```python
from build123d import *

# Parameters (mm, degrees)
EXTRUDE_THIN1_DEPTH       = 100
BOSS_EXTRUDE1_START       = -10
BOSS_EXTRUDE1_DEPTH       = 10
SKETCH3_R                 = 2.25
BOSS_EXTRUDE2_DEPTH       = 5
BOSS_EXTRUDE3_DEPTH       = 10
SKETCH5_R                 = 2.25
CUT_EXTRUDE1_DEPTH        = 6
BOSS_EXTRUDE4_REACH       = 121.416
BOSS_EXTRUDE4_END_RADIUS  = 39
SKETCH10_W                = 20
SKETCH10_H                = 20
BOSS_EXTRUDE5_START       = -29.189050103
BOSS_EXTRUDE5_OUTLINE_W   = 20
BOSS_EXTRUDE5_OUTLINE_H   = 20
BOSS_EXTRUDE5_DEPTH       = 29.189050103
BOSS_EXTRUDE5_START_2     = 80.604897745
BOSS_EXTRUDE5_2_OUTLINE_W = 23
BOSS_EXTRUDE5_2_OUTLINE_H = 23
BOSS_EXTRUDE5_2_DEPTH     = 1.395102255
BOSS_EXTRUDE6_DEPTH       = 20
SKETCH12_R                = 2.5
CUT_EXTRUDE2_DEPTH        = 20


with BuildPart() as part:
    # Sketch1 → Extrude-Thin1 (new body)
    with BuildSketch(Plane.XY):
        with BuildLine():
            ThreePointArc((-35, 0), (0, -35), (35, 0))
            Line((35, 0), (39, 0))
            ThreePointArc((39, 0), (0, -39), (-39, 0))
            Line((-39, 0), (-35, 0))
        make_face()
    extrude(amount=EXTRUDE_THIN1_DEPTH)

    # Sketch2 → Boss-Extrude1 (add)
    with BuildSketch(Plane.XY.offset(100).offset(BOSS_EXTRUDE1_START)):
        with BuildLine():
            Line((0, -39), (0, -35))
            Line((0, -35), (-10, -35))
            Line((-10, -35), (-10, -37.69615365))
            ThreePointArc((-10, -37.69615365), (-5.042321274, -38.672664715), (0, -39))
        make_face()
        with BuildLine():
            Line((10, -35), (0, -35))
            Line((0, -35), (0, -39))
            ThreePointArc((0, -39), (5.042321274, -38.672664715), (10, -37.69615365))
            Line((10, -37.69615365), (10, -35))
        make_face()
        with BuildLine():
            ThreePointArc((10, -37.69615365), (5.042321274, -38.672664715), (0, -39))
            ThreePointArc((0, -39), (-5.042321274, -38.672664715), (-10, -37.69615365))
            Line((-10, -37.69615365), (-10, -43))
            Line((-10, -43), (10, -43))
            Line((10, -43), (10, -37.69615365))
        make_face()
    extrude(amount=BOSS_EXTRUDE1_DEPTH)

    # Sketch3 → Boss-Extrude2 (add)
    with BuildSketch(Plane.XY.offset(100)):
        with Locations((-5, -39)):
            Circle(SKETCH3_R)
        with Locations((5, -39)):
            Circle(SKETCH3_R)
    extrude(amount=BOSS_EXTRUDE2_DEPTH)

    # Sketch4 → Boss-Extrude3 (add)
    with BuildSketch(Plane(origin=(0, 0, 0), x_dir=(-1, 0, 0), z_dir=(0, 0, -1))):
        with BuildLine():
            Line((0, -39), (0, -35))
            Line((0, -35), (-10, -35))
            Line((-10, -35), (-10, -37.69615365))
            ThreePointArc((-10, -37.69615365), (-5.042321274, -38.672664715), (0, -39))
        make_face()
        with BuildLine():
            ThreePointArc((10, -37.69615365), (5.042321274, -38.672664715), (0, -39))
            ThreePointArc((0, -39), (-5.042321274, -38.672664715), (-10, -37.69615365))
            Line((-10, -37.69615365), (-10, -43))
            Line((-10, -43), (10, -43))
            Line((10, -43), (10, -37.69615365))
        make_face()
        with BuildLine():
            Line((10, -35), (0, -35))
            Line((0, -35), (0, -39))
            ThreePointArc((0, -39), (5.042321274, -38.672664715), (10, -37.69615365))
            Line((10, -37.69615365), (10, -35))
        make_face()
    extrude(amount=-BOSS_EXTRUDE3_DEPTH)

    # Sketch5 → Cut-Extrude1 (cut)
    with BuildSketch(Plane(origin=(0, 0, 0), x_dir=(-1, 0, 0), z_dir=(0, 0, -1))):
        with Locations(Location((-5, -39, 0), (0, 0, 180))):
            Circle(SKETCH5_R)
        with Locations(Location((5, -39, 0), (0, 0, 180))):
            Circle(SKETCH5_R)
    extrude(amount=-CUT_EXTRUDE1_DEPTH, mode=Mode.SUBTRACT)

    # Boss-Extrude4: up to this cylinder (the profile starts outside it)
    boss_extrude4_end = Plane(origin=(0, 0, 50), z_dir=(0, 0, -1)) * Cylinder(BOSS_EXTRUDE4_END_RADIUS, 321.832, mode=Mode.PRIVATE)
    # Sketch10 → Boss-Extrude4 (add, up to the surface)
    with BuildSketch(Plane(origin=(0, -51.355775573, 4.493048169), x_dir=(1, 0, 0), z_dir=(0, 0.9961946980917462, -0.08715574274765152)), mode=Mode.PRIVATE) as boss_extrude4_sk1:
        with Locations((0, -45.680780994)):
            Rectangle(SKETCH10_W, SKETCH10_H)
    boss_extrude4_tool1 = extrude(boss_extrude4_sk1.sketch, amount=BOSS_EXTRUDE4_REACH, mode=Mode.PRIVATE) - boss_extrude4_end
    add(boss_extrude4_tool1.solids().sort_by_distance((0, -47.374433, 50))[0])

    # Boss-Extrude5: read off the stored shape, not the designer's step
    # Boss-Extrude5 outline → Boss-Extrude5 (add)
    with BuildSketch(Plane(origin=(0, -51.355775573, 4.493048169), x_dir=(1, 0, 0), z_dir=(0, 0.9961946980917462, -0.08715574274765152)).offset(BOSS_EXTRUDE5_START)):
        with Locations((0, -45.680780994)):
            Rectangle(BOSS_EXTRUDE5_OUTLINE_W, BOSS_EXTRUDE5_OUTLINE_H)
    extrude(amount=BOSS_EXTRUDE5_DEPTH)

    # Boss-Extrude5 2 outline → Boss-Extrude5 2 (cut)
    with BuildSketch(Plane(origin=(0, 0, 0), x_dir=(0.9994119135527714, 0.034137480457277325, -0.0032341114416132855), z_dir=(0.03429033462636031, -0.994956889147722, 0.09426007473315588)).offset(BOSS_EXTRUDE5_START_2)):
        with Locations((-2.5, 45.5)):
            Rectangle(BOSS_EXTRUDE5_2_OUTLINE_W, BOSS_EXTRUDE5_2_OUTLINE_H)
    extrude(amount=BOSS_EXTRUDE5_2_DEPTH, mode=Mode.SUBTRACT)

    # Sketch11 → Boss-Extrude6 (add, along a direction that is not the sketch's normal)
    with BuildSketch(Plane(origin=(10, 0, 0), x_dir=(0, 0, -1), z_dir=(1, 0, 0))):
        Polygon((-62.433599326, -74.753991325), (-42.522237652, -76.640350885), (-41.650680224, -66.678403904), (-61.562041898, -64.792044344), align=None)
    extrude(amount=BOSS_EXTRUDE6_DEPTH, dir=(0.999411883181242, 0.034160731366775, -0.002988676732389044))

    # Sketch12 → Cut-Extrude2 (cut)
    with BuildSketch(Plane(origin=(2.421276084, -70.254937612, 6.655801615), x_dir=(0.9994101830326217, 0.033961906388074226, -0.00508674406564492), z_dir=(-0.03429033462636031, 0.994956889147722, -0.09426007473315609))):
        with Locations(Location((17.489772292, -50.21182287, 0), (0, 0, 269.893376297))):
            Circle(SKETCH12_R)
        with Locations(Location((17.508382589, -40.211323595, 0), (0, 0, 269.893376297))):
            Circle(SKETCH12_R)
    extrude(amount=-CUT_EXTRUDE2_DEPTH, mode=Mode.SUBTRACT)


solid = part.part
```
Input: part model. Units: mm. Frame: model coordinates. A direction names the side the tool comes from. Round coordinates to 2 decimals unless told otherwise and drop trailing zeros. Order: outer loops, then holes, each group sorted by start corner. A loop starts at its lowest first (then second) coordinate and runs counter-clockwise, first axis right, second up. Notation, with made-up numbers: (4, 59.5) - (20, 59.5) arc R25 ccw to (20, 93.5) - close; hole circle Ø8 at (-40, 48.25). An arc over 180 degrees is marked (long way). One line per question, with ' | ' between items. Start each with the question number.
1) Pull-direction query (X, two-part tool) for faces 6 (the flat face through (10, -40, 5)), 7 (the cylindrical face through (-5.29, -36.77, 102.46)), 8 (the flat face through (0, -43, 5)), 9 (the cylindrical face through (-12.53, -36.932, 49.3)); classes: +X half, -X half, draft (parallel to the pull), parting line (faces both ways), or undercut.
2) Cut plane D-D, the plane z = 13.5. Return the cut outline in (x, y), then the cut area to 3 significant figures.
3) Cut plane B-B, the plane z = 95. Return the cut outline in (x, y), then the cut area to 3 significant figures.
4) Contact query for flat-ended pins moving along their axis: P1, Ø2.5, axis at y = -39, z = 96, coming from the +X side; P2, Ø6, axis at x = -29, z = 48, coming from the +Y side; P3, Ø4, axis at x = 5, y = -39, coming from the -Z side. Output: stop coordinate, or through.
5) Set-up query: faces 1 (the flat face through (-5, -39, 105)), 2 (the cylindrical face through (-0.77, -34.99, 49.3)), 3 (the flat face through (-5, -39, 6)), 4 (the cylindrical face through (4.71, -36.77, 102.46)), 5 (the flat face through (10, -40, 95)). Return all of +Z, -Z, +X, -X, +Y, -Y with unobstructed straight access to the full face (end or side cutting, diameter ignored); none if empty.
6) Cut plane A-A, the plane y = -11. Return the cut outline in (x, z).
7) Cut plane C-C, the plane x = 0. Return the cut outline in (y, z).
8) Ray query, probe 1 along X at (y, z) = (-39, 4); probe 2 along Y at (x, z) = (-5, 2); probe 3 along Z at (x, y) = (-34.5, -7.5). Return the intervals inside material, ascending.
Worked out:
1) face 6: +X half | face 7: undercut | face 8: draft | face 9: parting line
2) outline: (-39, 0) arc R39 ccw to (39, 0) - (35, 0) arc R35 cw to (-35, 0) - close | area: 465 mm^2
3) outline: (-39, 0) arc R39 ccw to (-10, -37.7) - (-10, -43) - (10, -43) - (10, -37.7) arc R39 ccw to (39, 0) - (35, 0) arc R35 cw to (-35, 0) - close | area: 554 mm^2
4) P1: stops at x = 10 | P2: stops at y = -14.18 | P3: stops at z = 6
5) face 1: +Z, +X, -X, +Y, -Y | face 2: +Z, -Z, +Y | face 3: -Z | face 4: +Z | face 5: +Z, -Z, +X, -Y
6) outline: (-37.42, 0) - (-33.23, 0) - (-33.23, 100) - (-37.42, 100) - close; (33.23, 0) - (37.42, 0) - (37.42, 100) - (33.23, 100) - close
7) outline: (-76.98, 42.55) - (-39, 39.23) - (-39, 10) - (-43, 10) - (-43, 0) - (-35, 0) - (-35, 100) - (-43, 100) - (-43, 90) - (-39, 90) - (-39, 59.31) - (-75.1, 62.46) - close
8) probe 1: x = -10 to -7.25, -2.75 to 2.75, 7.25 to 10 | probe 2: y = -43 to -41.25, -36.75 to -34.64 | probe 3: z = 0 to 100
